from build123d import *

# Parameters (mm, degrees)
F2_DEPTH = 25.4
F4_DEPTH = 9.906
F6_DEPTH = 1.016


# Not quite as in the source:
# - the program builds the solid bodies; features that only make, move or delete a surface that nothing else refers to are left out


with BuildPart() as f2:
    # F0 (on Top) → F2 (new body)
    with BuildSketch(Plane.XY):
        Polygon((-98.1804851865, 42.2748850128), (-83.6932088757, 12.0514331916), (-50.2752936531, 9.4860565979), (-31.3446547413, 37.1441318253), (-45.8319310522, 67.3675836465), (-79.2498462748, 69.9329602402), align=None)
    extrude(amount=F2_DEPTH)

    # F4 (cut): a face of the model
    f4_faces = [f2.faces().sort_by_distance(p)[0] for p in [
        (-62.5408886635, 68.6502719433, 12.7),
    ]]
    extrude(f4_faces, amount=-F4_DEPTH, mode=Mode.SUBTRACT)

    # F5 (on Top) → F6 (join)
    with BuildSketch(Plane.XY):
        with BuildLine():
            add(Edge.make_bspline(
                [(-63.3374005556, 107.8479960561), (-90.0996928702, 107.8479960561), (-76.7185467129, 70.8282925189), (-63.3374005556, 33.8085889816), (-49.9562543983, 70.8282925189), (-36.575108241, 107.8479960561), (-63.3374005556, 107.8479960561)],
                knots=[0, 0, 0, 2.0943951024, 2.0943951024, 4.1887902048, 4.1887902048, 6.2831853072, 6.2831853072, 6.2831853072], degree=2, weights=[1, 0.5, 1, 0.5, 1, 0.5, 1]))
        make_face()
    extrude(amount=-F6_DEPTH)


solid = f2.part
CAD build for the part. Positions are in the model's coordinates, mm. A direction names the side the tool comes from. Round coordinates to 2 decimals unless told otherwise and drop trailing zeros. Loops run counter-clockwise (first coordinate to the right, second up) from the corner with the lowest first, then second, coordinate; pieces in that order, holes last. Notation, with made-up numbers: M 75.5,23 L 105.5,23 A31 ccw 105.5,59 Z; hole C 39,38.25 d11. An arc over 180 degrees is marked long. One line per question, with ' | ' between items. Start each with the question number.
Item 1: Pin check, flat tips, straight feed: pin 1 Ø4 at (x, y) = (-84, 22) entering from -Z; pin 2 Ø8 at (x, z) = (-66, 20) entering from +Y; pin 3 Ø6 at (x, z) = (-57, 12) entering from -Y. Stop position of each tip, or through.
Item 2: Cut at A-A, the plane z = 7. Write the cut outline in (x, y), plus the area to 3 significant figures.
Item 3: Cut at C-C, the plane x = -44. Write the cut outline in (y, z).
Item 4: Two-plate mould, pull along Y, no slides. Class faces 4 (the flat face through (-88.58, 56.3, 12.52)), 5 (the flat face through (-79.624, 65.064, 12.522)), 6 (the flat face through (-65, 40, 25.4)), 7 (the flat face through (-40.942, 23.121, 12.522)): pulls with the +Y half, pulls with the -Y half, needs draft (parallel to the pull), parting line crosses it, or undercut.
Item 5: Which spindle directions (+Z, -Z, +X, -X, +Y, -Y) get a long thin tool onto all of the face, cutting with end or side? Do faces 1 (the flat face through (-46.206, 62.498, 12.522)), 2 (the flat face through (-67.218, 10.787, 12.522)), 3 (the flat face through (-64, 84, 0)). Say none if no direction does.
Item 6: Wall check: line 1 (Z direction, x = -52.5, y = 88); line 2 (Z direction, x = -75.5, y = 47); line 3 (Y direction, x = -91.5, z = 16). Give the ranges that are in metal, low to high.
Item 7: Cut at B-B, the plane y = 65. State how many separate pieces and enclosed holes the cut face has, plus the area to 3 significant figures.
Item 8: Cut at D-D, the plane y = 50.5. Write the cut outline in (x, z), plus the area to 3 significant figures.
Responses:
1) pin 1: stops at z = 0 | pin 2: stops at y = 59.29 | pin 3: stops at y = 9.77
2) outline: M -98.18,42.27 L -83.69,12.05 L -50.28,9.49 L -31.34,37.14 L -45.83,67.37 L -46.59,57.49 L -80.01,60.06 L -79.25,69.93 Z | area: 2,590 mm²
3) outline: M 18.65,0 L 63.55,0 L 63.55,25.4 L 18.65,25.4 Z
4) face 4: pulls with the +Y half | face 5: undercut | face 6: needs draft | face 7: pulls with the -Y half
5) face 1: +Z, -Z, +Y | face 2: +Z, -Z, -X, -Y | face 3: +Z, +Y
6) line 1: z = -1.02 to 0 | line 2: z = 0 to 25.4 | line 3: y = 28.34 to 52.04
7) separate pieces: 3 | enclosed holes: 0 | area: 131 mm²
8) outline: M -92.55,0 L -37.75,0 L -37.75,25.4 L -92.55,25.4 Z | area: 1,390 mm²
